```python
from build123d import *

# Parameters (mm, degrees)
F0_W     = 10
F0_H     = 18
F1_DEPTH = 1.75
F2_W     = 10
F2_H     = 1.75
F2_H_2   = 5.2
F3_DEPTH = 2
F8_R     = 0.5
F9_R     = 1.24999


# Not quite as in the source:
# - a fillet or chamfer is up to 0.001 mm smaller than in the source, because OpenCascade refuses the exact size


with BuildPart() as f1:
    # F0 (on Top) → F1 (new body)
    with BuildSketch(Plane.XY):
        Rectangle(F0_W, F0_H)
    extrude(amount=F1_DEPTH)

    # F2 (on face) → F3 (join)
    with BuildSketch(Plane(origin=(0, 9, 0), x_dir=(-1, 0, 0), z_dir=(0, 1, 0))):
        with Locations((0, 0.875)):
            Rectangle(F2_W, F2_H)
        with Locations((0, -2.6)):
            Rectangle(F2_W, F2_H_2)
    extrude(amount=F3_DEPTH)

    # F7: F1 across plane


with BuildPart() as f1_1:
    add(f1.part)
    add(f1.part.mirror(Plane(origin=(-5, 1.2789499015, -1.725), x_dir=(0.9979743188, 0.063618071, 0), z_dir=(0, 0, -1))))

    # F8
    f8_edges = [f1_1.edges().sort_by_distance(p)[0] for p in [
        (0, 9, 0),
        (0, 9, -3.45),
        (5, 0, -3.45),
        (-5, 0, -3.45),
        (0, -9, -3.45),
        (5, 0, 0),
        (-5, 0, 0),
        (0, -9, 0),
        (5, 9, -1.725),
        (-5, 9, -1.725),
    ]]
    fillet(f8_edges, radius=F8_R)

    # F9 (radius 1.25 in the source; OpenCascade refuses exactly that, so slightly less here)
    f9_edges = [f1_1.edges().sort_by_distance(p)[0] for p in [
        (5, 11, -1.725),
        (0, 11, -5.2),
        (-5, 11, -1.725),
        (0, 11, 1.75),
        (5, 1, 1.75),
        (-5, 1, 1.75),
        (0, -9, 1.75),
        (-5, 1, -5.2),
        (0, -9, -5.2),
        (5, 1, -5.2),
    ]]
    fillet(f9_edges, radius=F9_R)


solid = f1_1.part
```
Could you check a few things on this model? Use its own coordinates, in mm. A direction names the side the tool comes from. Round coordinates to 2 decimals unless told otherwise and drop trailing zeros. Order: outer loops, then holes, each group sorted by start corner. A loop starts at its lowest first (then second) coordinate and runs counter-clockwise, first axis right, second up. Notation, with made-up numbers: M 9.5,3.25 L 48.5,3.25 A21 cw 48.5,9.25 Z; hole C -5,87.5 d1. An arc over 180 degrees is marked long. One line per question, with ' | ' between items. Start each with the question number.
(1) Please list where these lines run through material, in increasing order: line 1 along Z through (x, y) = (2.25, 0.75); line 2 along X through (y, z) = (-6.5, -4); line 3 along Y through (x, z) = (1.25, -4).
(2) Thinking about a two-plate mould opening in Z: for faces 3 (the face through (0.07, -8.624, 1.394)), 4 (the face through (0, 9, -2)), 5 (the face through (0, 1, -5.2)), which applies, +Z half, -Z half, draft (parallel to the pull), parting line (faces both ways), or undercut?
(3) Suppose I cut it at B-B on z = -1.25. List the corners of the cut face in (x, y) for me.
(4) For faces 1 (the face through (-4.624, 0.244, 1.394)), 2 (the face through (0, 0, -3.45)), which set-ups out of +Z, -Z, +X, -X, +Y, -Y let a thin tool reach every point of the face, with its end or its side?
(5) For P1, Ø2, axis at x = 1, z = -2, coming from the -Y side, with a flat end and sliding along its axis, tell me the tip position at first contact or that it passes through.
Geometry results:
1) line 1: -5.2 to -3.45, 0 to 1.75 | line 2: -5 to 5 | line 3: -9 to 11
2) face 3: +Z half | face 4: undercut | face 5: -Z half
3) outline: M -5,9.5 A0.5 ccw -4.5,9 L 4.5,9 A0.5 ccw 5,9.5 L 5,9.75 A1.25 ccw 3.75,11 L -3.75,11 A1.25 ccw -5,9.75 Z
4) face 1: +Z, -X, +Y, -Y | face 2: +X, -X, -Y
5) P1: y = 9
